from build123d import *

# Parameters (mm, degrees)
SKETCH1_R                       = 6.55
BOSS_EXTRUDE1_DEPTH             = 7
CHAMFER1_SIZE                   = 1
FILLET1_R                       = 2
F_3_0MM_DOWEL_HOLE1_D           = 3
F_3_0MM_DOWEL_HOLE1_CSINK_D     = 3.05
F_3_0MM_DOWEL_HOLE1_CSINK_ANGLE = 90


with BuildPart() as part:
    # Sketch1 → Boss-Extrude1 (new body)
    with BuildSketch(Plane.XY):
        with BuildLine():
            Line((-9, 0), (-9, -10))
            Line((-9, -10), (-16.5, -22.990381057))
            Line((-16.5, -22.990381057), (-7.5, -38.578838325))
            Line((-7.5, -38.578838325), (9, -10))
            Line((9, -10), (9, 0))
            ThreePointArc((9, 0), (0, 9), (-9, 0))
        make_face()
        Circle(SKETCH1_R, mode=Mode.SUBTRACT)
    extrude(amount=BOSS_EXTRUDE1_DEPTH)

    # Chamfer1
    chamfer1_edges = [part.edges().sort_by_distance(p)[0] for p in [
        (-6.55, 0, 0),
        (-6.55, 0, 7),
    ]]
    chamfer(chamfer1_edges, length=CHAMFER1_SIZE)

    # Fillet1
    fillet1_edges = [part.edges().sort_by_distance(p)[0] for p in [
        (9, -10, 3.5),
        (-7.5, -38.578838325, 3.5),
        (-16.5, -22.990381057, 3.5),
        (-9, -10, 3.5),
    ]]
    fillet(fillet1_edges, radius=FILLET1_R)

    # Ø3.0mm Dowel Hole1 (through all)
    with Locations(Plane.XY.offset(7)):
        with Locations((-11.303847577, -21.990381057), (-6.803847577, -29.784609691), (-2.303847577, -21.990381057)):
            CounterSinkHole(F_3_0MM_DOWEL_HOLE1_D / 2, F_3_0MM_DOWEL_HOLE1_CSINK_D / 2, counter_sink_angle=F_3_0MM_DOWEL_HOLE1_CSINK_ANGLE)


solid = part.part
For this review, take the finished solid that the model builds, in its own axes (mm). A direction names the side the tool comes from. Round coordinates to 2 decimals unless told otherwise and drop trailing zeros. Write each loop counter-clockwise with the first axis right and the second up, starting at its lowest first coordinate (ties: lowest second). Pieces come first, ordered by that corner, then holes. Notation, with made-up numbers: (-19, 41.25) -> (28, 41.25) arc R23 ccw to (28, 63.25) -> close; hole circle Ø7 at (22.5, -28). An arc over 180 degrees is marked (long way). Use CSV: the item, a comma, the result in double quotes.
(1) To check wall thickness, follow L1, parallel to Y at x = -1.25, z = 1.25; L2, parallel to Y at x = -5.75, z = 4; L3, parallel to X at y = -9, z = 1. State the ranges of each line that lie inside material, in increasing order. Write a range as [from, to].
Computed values:
L1,"[-27.75, -23.06], [-20.92, -6.43], [6.43, 8.91]"
L2,"[-35.55, -30.85], [-28.72, -3.14], [3.14, 6.92]"
L3,"[-9, 9]"
(2) For faces 4 (the face through (-12.624, -29.703, 3.451)), 5 (the face through (-9, -5, 3)), list the 3-axis set-ups (+Z, -Z, +X, -X, +Y, -Y) from which the entire face can be reached by the end or side of a thin tool; tool diameter is ignored.
Computed values:
face 4,"+Z, -Z, -X, -Y"
face 5,"+Z, -Z, -X, +Y"
(3) Consider section B-B, the plane z = 5.5. Give the boundary of the cut face in (x, y).
Computed values:
outline,"(-15.92, -23.99) -> (-9.23, -35.58) arc R2 ccw to (-5.77, -35.58) -> (8.73, -10.46) arc R2 ccw to (9, -9.46) -> (9, 0) arc R9 ccw to (-9, 0) -> (-9, -9.46) arc R2 cw to (-9.27, -10.46) -> (-15.92, -21.99) arc R2 ccw to start; hole circle Ø3 at (-11.3, -21.99); hole circle Ø3 at (-6.8, -29.78); hole circle Ø13.1 at (0, 0); hole circle Ø3 at (-2.3, -21.99)"
(4) Consider section A-A, the plane x = 0. Give the boundary of the cut face in (y, z).
Computed values:
outline,"(-25.59, 0) -> (-7.55, 0) -> (-6.55, 1) -> (-6.55, 6) -> (-7.55, 7) -> (-25.59, 7) -> close; (6.55, 1) -> (7.55, 0) -> (9, 0) -> (9, 7) -> (7.55, 7) -> (6.55, 6) -> close"
(5) Clearance check with flat-ended pins moving along their axes: P1, Ø1.8, axis at x = -6.8, y = -29.78, coming from the +Z side; P2, Ø2, axis at y = -3, z = 3, coming from the -X side; P3, Ø3, axis at y = -20.5, z = 1, coming from the -X side; P4, Ø2, axis at x = -10.5, z = 6, coming from the -Y side. State where each tip first meets the part, or that it passes through.
Computed values:
P1,"through"
P2,"x = -9"
P3,"x = -15.93"
P4,"y = -35.11"
(6) Consider section C-C, the plane y = -20. Give the boundary of the cut face in (x, z), plus the area to 3 significant figures.
Computed values:
outline,"(-14.77, 0) -> (3.23, 0) -> (3.23, 7) -> (-14.77, 7) -> close"
area,"126 mm²"
(7) Draft analysis for pull direction Y (two halves, no side actions). For faces 1 (the face through (-4, -13, 0)), 2 (the face through (0, 9, 3)), 3 (the face through (-1.979, -23.455, 3.439)), state which applies: +Y half, -Y half, draft (parallel to the pull), parting line (faces both ways), or undercut.
Computed values:
face 1,"draft"
face 2,"+Y half"
face 3,"undercut"
